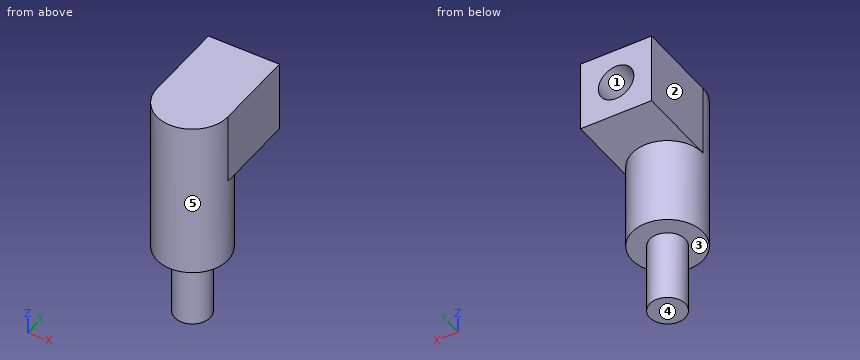
```python
from build123d import *

# Parameters (mm, degrees)
SKETCH1_LINK4_R     = 15
BOSS_EXTRUDE1_DEPTH = 30
SKETCH2_LINK4_R     = 30
BOSS_EXTRUDE2_DEPTH = 73.3
BOSS_EXTRUDE3_DEPTH = 60
SKETCH4_LINK4_R     = 15
CUT_EXTRUDE1_DEPTH  = 30


with BuildPart() as part:
    # sketch1_link4 → Boss-Extrude1 (new body, symmetric)
    with BuildSketch(Plane.XY):
        Circle(SKETCH1_LINK4_R)
    extrude(amount=BOSS_EXTRUDE1_DEPTH, both=True)

    # sketch2_link4 → Boss-Extrude2 (add)
    with BuildSketch(Plane.XY.offset(30)):
        Circle(SKETCH2_LINK4_R)
    extrude(amount=BOSS_EXTRUDE2_DEPTH)

    # sketch3_link4 → Boss-Extrude3 (add)
    with BuildSketch(Plane.XY.offset(103.3)):
        with BuildLine():
            Line((-30, 0), (-30, 69.7))
            Line((-30, 69.7), (30, 69.7))
            Line((30, 69.7), (30, 0))
            ThreePointArc((30, 0), (0, -30), (-30, 0))
        make_face()
    extrude(amount=BOSS_EXTRUDE3_DEPTH)

    # sketch4_link4 → Cut-Extrude1 (cut)
    with BuildSketch(Plane(origin=(0, 69.7, 0), x_dir=(1, 0, 0), z_dir=(0, 1, 0))):
        with Locations((0, -133.3)):
            Circle(SKETCH4_LINK4_R)
    extrude(amount=-CUT_EXTRUDE1_DEPTH, mode=Mode.SUBTRACT)


solid = part.part
```
For this review, take the finished solid that the model builds, in its own axes (mm). Face numbers are marked on the shaded views. A direction names the side the tool comes from. Coordinates: 2 decimals unless noted, no trailing zeros. Loops run counter-clockwise (first coordinate to the right, second up) from the corner with the lowest first, then second, coordinate; pieces in that order, holes last. Notation, with made-up numbers: (26, 16.5) -> (44, 16.5) arc R25 cw to (44, 33.5) -> close; hole circle Ø2 at (-15, 45.5). An arc over 180 degrees is marked (long way). Return JSON: item names as keys, results as strings. Group by question number.
(1) Consider section B-B, the plane y = 46. Give the boundary of the cut face in (x, z), plus the area to 3 significant figures.
(2) For pin 1 Ø3 at (x, z) = (5, 97.5) entering from -Y; pin 2 Ø24 at (x, z) = (0, 133.3) entering from -Y; pin 3 Ø4 at (x, y) = (-2, 19.5) entering from -Z, all flat-tipped, find the tip position at first contact; note any pin that passes through.
(3) Mouldability with a two-part tool opening along X and no side actions: class the marked faces 1, 2 and 3 as pulls with the +X half, pulls with the -X half, needs draft (parallel to the pull), parting line crosses it, or undercut.
(4) Consider section C-C, the plane x = 0. Give the boundary of the cut face in (y, z).
(5) Consider section A-A, the plane z = 133.3. Give the boundary of the cut face in (x, y).
(6) Consider section D-D, the plane y = 2. Give the boundary of the cut face in (x, z), plus the area to 3 significant figures.
(7) To check wall thickness, follow L1, parallel to X at y = 57, z = 133; L2, parallel to Z at x = 0, y = 57.25; L3, parallel to Y at x = 1, z = 50.5. State the ranges of each line that lie inside material, in increasing order.
(8) Tool access review of the marked faces 4 and 5: name each direction out of +Z, -Z, +X, -X, +Y, -Y from which nothing blocks a thin tool from reaching the whole face with its end or side.
Results below:
{
 "1": {"outline": "(-30, 103.3) -> (30, 103.3) -> (30, 163.3) -> (-30, 163.3) -> close; hole circle Ø30 at (0, 133.3)", "area": "2,890 mm2"},
 "2": {"pin 1": "stops at y = -29.8", "pin 2": "stops at y = -30", "pin 3": "stops at z = 30"},
 "3": {"face 1": "undercut", "face 2": "pulls with the -X half", "face 3": "needs draft"},
 "4": {"outline": "(-30, 30) -> (-15, 30) -> (-15, -30) -> (15, -30) -> (15, 30) -> (30, 30) -> (30, 103.3) -> (69.7, 103.3) -> (69.7, 118.3) -> (39.7, 118.3) -> (39.7, 148.3) -> (69.7, 148.3) -> (69.7, 163.3) -> (-30, 163.3) -> close"},
 "5": {"outline": "(-30, 0) arc R30 ccw to (30, 0) -> (30, 69.7) -> (15, 69.7) -> (15, 39.7) -> (-15, 39.7) -> (-15, 69.7) -> (-30, 69.7) -> close"},
 "6": {"outline": "(-30, 103.3) -> (-29.93, 103.3) -> (-29.93, 30) -> (-14.87, 30) -> (-14.87, -30) -> (14.87, -30) -> (14.87, 30) -> (29.93, 30) -> (29.93, 103.3) -> (30, 103.3) -> (30, 163.3) -> (-30, 163.3) -> close", "area": "9,770 mm2"},
 "7": {"L1": "x = -30 to -15, 15 to 30", "L2": "z = 103.3 to 118.3, 148.3 to 163.3", "L3": "y = -29.98 to 29.98"},
 "8": {"face 4": "-Z, +X, -X, +Y, -Y", "face 5": "-Z"}
}
